Autodesk Inventor part; units mm, degrees
ref_plane "XZ Plane" through (0, 0, 0) normal (0, 1, 0) x (-1, 0, 0)
ref_plane "XY Plane" through (0, 0, 0) normal (0, 0, 1) x (1, 0, 0)
sketch "Szkic1" plane through (0, 0, 0) normal (0, 0, 1) x (1, 0, 0)
  line L0 (0, 0) -> (37, 0)
  line L1 (37, 0) -> (37, 22)
  line L2 (37, 22) -> (0, 22)
  line L3 (0, 11) -> (-5, 11) construction
  circle A0 centre (-2, 11) radius 1.25
  arc A1 (0, 16) -> (0, 6) centre (0, 11) ccw
  line L4 (37, 22) -> (32, 22) construction
  line L5 (37, 22) -> (37, 19.5) construction
  circle A2 centre (32, 19.5) radius 1.5
  line L6 (37, 0) -> (32, 0) construction
  line L7 (32, 0) -> (32, 2.5) construction
  circle A3 centre (32, 2.5) radius 1.5
  line L8 (0, 22) -> (37, 22)
  line L9 (37, 22) -> (37, 25)
  line L10 (37, 25) -> (0, 25)
  line L11 (0, 25) -> (0, 22)
  line L12 (0, 0) -> (37, 0)
  line L13 (37, 0) -> (37, -3)
  line L14 (37, -3) -> (0, -3)
  line L15 (0, -3) -> (0, 0)
  line L16 (0, 22) -> (0, 16)
  line L17 (0, 6) -> (0, 0)
  dimension "d0" = 37
  dimension "d1" = 22
  dimension "d2" = 5
  dimension "d3" = 2.5
  dimension "d7" = 3
  dimension "d10" = 3
  dimension "d11" = 37
  dimension "d12" = 3
  dimension "d13" = 37
  dimension "d14" = 3
extrude "Wyciągnięcie proste1" add sketch "Szkic1" along normal blind 4 contours L17 A1 L16 L2 L1 L0
sketch "Szkic2" plane through (0, 0, 4) normal (0, 0, 1) x (1, 0, 0)
  circle A0 centre (-2, 11) radius 1.25
  arc A1 (0, 16) -> (0, 6) centre (0, 11) ccw
  line L0 (0, 6) -> (0, 0)
  line L1 (0, 16) -> (0, 6)
extrude "Wyciągnięcie proste2" add sketch "Szkic2" along normal blind 3
extrude "Wyciągnięcie proste3" add sketch "Szkic1" along normal blind 19 contours L0 L13 L14 L15
extrude "Wyciągnięcie proste4" add sketch "Szkic1" along normal blind 19 contours L2 L11 L10 L9
fillet "Zaokrąglenie2" radius 1.5 1 edges at (18.5, 25, 19)
fillet "Zaokrąglenie3" radius 1.5 1 edges at (18.5, -3, 19)
sketch "Szkic3" plane through (0, 25, 0) normal (0, 1, 0) x (1, 0, 0)
  line L0 (37, -17.5) -> (0, -17.5)
  line L1 (37, 0) -> (37, -17.5)
  line L2 (37, 0) -> (0, 0)
  line L3 (0, 0) -> (0, -17.5)
  line L4 (-5, 0) -> (0, 0)
  line L5 (0, 0) -> (37, 0)
  line L6 (37, 0) -> (37, -5)
  line L7 (37, -5) -> (0, -5)
  line L8 (0, -5) -> (0, 0)
  dimension "d26" = 37
  dimension "d27" = 5
extrude "Wyciągnięcie proste5" add sketch "Szkic3" along normal blind 9 contours L7 L3 L2 L1
sketch "Szkic4" plane through (0, 25, 5) normal (0, 0, 1) x (1, 0, 0)
  line L0 (0, 9) -> (0, 0)
  line L1 (0, 0) -> (0, 4.5)
  line L2 (37, 0) -> (37, 9)
  circle A0 centre (6, 4.5) radius 1.5
  circle A1 centre (18.5, 4.5) radius 1.5
  circle A2 centre (30.5, 4.5) radius 1.5
  point P0 (0, -25)
  dimension "d30" = 3
  dimension "d31" = 3
  dimension "d32" = 3
extrude "Wyciągnięcie proste6" cut sketch "Szkic4" against normal blind 9
mirror "Odbij1" about plane through (37, 0, 0) normal (1, 0, 0)
ref_plane "Płaszczyzna konstrukcyjna1" through (37, 0, 0) normal (1, 0, 0) x (0, 1, 0)
split "Podział1" plane through (37, 0, 0) removes the side toward (-1, 0, 0)
sketch "Szkic5" plane through (37, 25, 5) normal (0, 0, 1) x (1, 0, 0)
  point P0 (-37, -25)
sketch "Szkic6" plane through (37, 34, 0) normal (0, 1, 0) x (1, 0, 0)
  point P0 (-37, 0)
sketch "Szkic7" plane through (74, -3, 0) normal (0, 0, -1) x (-1, 0, 0)
  point P0 (74, 3)
sketch "Szkic8" plane through (37, 34, 0) normal (0, 1, 0) x (1, 0, 0)
  point P0 (-37, 0)
sketch "Szkic9" plane through (37, 25, 5) normal (0, 0, 1) x (1, 0, 0)
  point P0 (-37, -25)
properties part number "motor_grip_L"
Could you check a few things on this model? Use its own coordinates, in mm. A direction names the side the tool comes from. Round coordinates to 2 decimals unless told otherwise and drop trailing zeros. Order: outer loops, then holes, each group sorted by start corner. A loop starts at its lowest first (then second) coordinate and runs counter-clockwise, first axis right, second up.
(1) I'm going to push flat-ended pins straight in: pin 1 (4 mm diameter, centred on y = 24, z = 13.5, fed in from +X); pin 2 (10 mm diameter, centred on y = 3, z = 5.5, fed in from +X); pin 3 (2.5 mm diameter, centred on y = 10, z = 5.5, fed in from -X); pin 4 (2.5 mm diameter, centred on x = 42, y = 19.5, fed in from -Z). Where does each tip first touch, or does it pass through?
Response values:
pin 1: stops at x = 74
pin 2: stops at x = 78
pin 3: stops at x = 74
pin 4: passes through
(2) Imagine slicing it at C-C (y = 11). Write out the boundary of the cut face in (x, z).
Response values:
outline: (37, 0) - (74.75, 0) - (74.75, 7) - (74, 7) - (74, 4) - (37, 4) - close; (77.25, 0) - (79, 0) - (79, 7) - (77.25, 7) - close
(3) Which directions (+Z, -Z, +X, -X, +Y, -Y) give clear straight access to the entire face, cutting with the end or side of a thin tool? Please do faces 1 (the flat face through (74, 11, 5)), 2 (the flat face through (74, -0.4, 7.3)), 3 (the flat face through (56, 22, 11)), 4 (the flat face through (56, 27, 5)), 5 (the cylindrical face through (66.57, 29.05, 2.54)).
Response values:
face 1: +Z, -X
face 2: +Z, -Z, +X, -Y
face 3: +Z, +X, -X
face 4: +Z, +X, -X, +Y
face 5: +Z, -Z
(4) Imagine slicing it at B-B (x = 55.5). Write out the boundary of the cut face in (y, z), plus the area to 3 significant figures.
Response values:
outline: (-3, 0) - (28, 0) - (28, 5) - (25, 5) - (25, 17.5) arc R1.5 ccw to (23.5, 19) - (22, 19) - (22, 4) - (0, 4) - (0, 19) - (-1.5, 19) arc R1.5 ccw to (-3, 17.5) - close; (31, 0) - (34, 0) - (34, 5) - (31, 5) - close
area: 231 mm2
(5) Imagine slicing it at D-D (z = 15.75). Write out the boundary of the cut face in (x, y).
Response values:
outline: (37, -3) - (74, -3) - (74, 0) - (37, 0) - close; (37, 22) - (74, 22) - (74, 25) - (37, 25) - close
(6) Please list where these lines run through material, in increasing order: line 1 along Y through (x, z) = (68, 2.9); line 2 along Y through (x, z) = (40, 16.5); line 3 along Z through (x, y) = (66, 19).
Response values:
line 1: y = -3 to 28, 31 to 34
line 2: y = -3 to 0, 22 to 25
line 3: z = 0 to 4
(7) If we mould it in two halves opening along X, with no side actions, what happens to faces 6 (the flat face through (74, 23, 5)), 7 (the flat face through (55, 0, 11)), 8 (the cylindrical face through (43.11, 20.51, 1.97)), 9 (the cylindrical face through (43.5, 2.57, 1.97))? For each: released by +X, released by -X, zero draft, split by the parting line, or undercut.
Response values:
face 6: released by +X
face 7: zero draft
face 8: undercut
face 9: undercut
(8) Imagine slicing it at A-A (z = 5.5). Write out the boundary of the cut face in (x, y), plus the area to 3 significant figures.
Response values:
outline: (37, -3) - (74, -3) - (74, 0) - (37, 0) - close; (37, 22) - (74, 22) - (74, 25) - (37, 25) - close; (74, 6) arc R5 ccw to (74, 16) - close; hole circle Ø2.5 at (76, 11)
area: 256 mm2
